Source: three-view drawing plus pictorial views. Frame: mm from the lowest corner of the part. Round coordinates to 2 decimals unless told otherwise and drop trailing zeros. Write each loop counter-clockwise with the first axis right and the second up, starting at its lowest first coordinate (ties: lowest second). Pieces come first, ordered by that corner, then holes. Notation, with made-up numbers: M 9,68 L 63,68 A19 ccw 63,84 Z; hole C -34,-21 d6. An arc over 180 degrees is marked long. Answer in a Markdown table with one row per item.
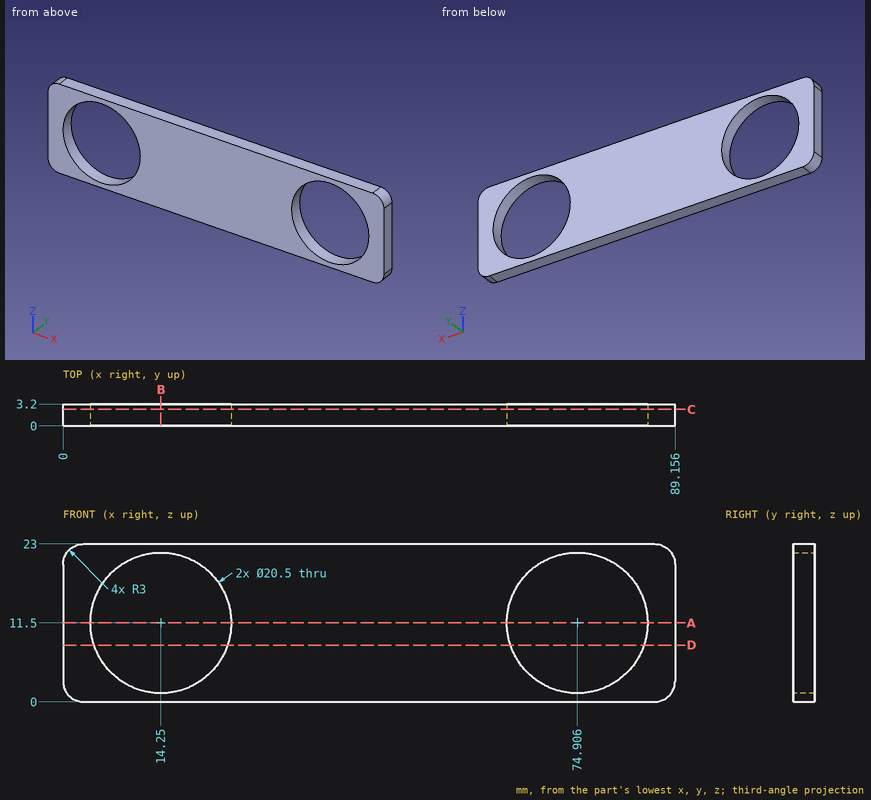
Q1. Section B-B (x = 14.25). Return loops of the section in (y, z).
Solutions:
| item | result |
|---|---|
| outline | M 0,0 L 3.2,0 L 3.2,1.25 L 0,1.25 Z; M 0,21.75 L 3.2,21.75 L 3.2,23 L 0,23 Z |
Q2. Material intervals for probe 1 along X at (y, z) = (1.75, 11.5); probe 2 along X at (y, z) = (2.5, 6.5), sorted ascending.
Solutions:
| item | result |
|---|---|
| probe 1 | x = 0 to 4, 24.5 to 64.66, 85.16 to 89.16 |
| probe 2 | x = 0 to 5.3, 23.2 to 65.96, 83.85 to 89.16 |
Q3. Contact query for a flat-ended pin moving along its axis: pin 1 Ø3 at (x, z) = (68.5, 15) entering from +Y. Output: stop coordinate, or through.
Solutions:
| item | result |
|---|---|
| pin 1 | passes through |
Q4. Section C-C (y = 2.4). Return loops of the section in (x, z), and give its area (3 significant figures).
Solutions:
| item | result |
|---|---|
| outline | M 0,3 A3 ccw 3,0 L 86.16,0 A3 ccw 89.16,3 L 89.16,20 A3 ccw 86.16,23 L 3,23 A3 ccw 0,20 Z; hole C 14.25,11.5 d20.5; hole C 74.91,11.5 d20.5 |
| area | 1,380 mm2 |
Q5. Section D-D (z = 8.25). Return loops of the section in (x, y), and give its area (3 significant figures).
Solutions:
| item | result |
|---|---|
| outline | M 0,0 L 4.53,0 L 4.53,3.2 L 0,3.2 Z; M 23.97,0 L 65.18,0 L 65.18,3.2 L 23.97,3.2 Z; M 84.63,0 L 89.16,0 L 89.16,3.2 L 84.63,3.2 Z |
| area | 161 mm2 |
Q6. Section A-A (z = 11.5). Return loops of the section in (x, y), and give its area (3 significant figures).
Solutions:
| item | result |
|---|---|
| outline | M 0,0 L 4,0 L 4,3.2 L 0,3.2 Z; M 24.5,0 L 64.66,0 L 64.66,3.2 L 24.5,3.2 Z; M 85.16,0 L 89.16,0 L 89.16,3.2 L 85.16,3.2 Z |
| area | 154 mm2 |
